Check sheet for the modelled part. Datum: model origin and axes. Units: mm. A direction names the side the tool comes from. Round coordinates to 2 decimals unless told otherwise and drop trailing zeros. Write each loop counter-clockwise with the first axis right and the second up, starting at its lowest first coordinate (ties: lowest second). Pieces come first, ordered by that corner, then holes.
Item 1: Release check for a two-part mould opening along Z. For faces 6 (the cylindrical face through (-27.101, 13.479, 31.486)), 7 (the flat face through (-40, 6, 24)), 8 (the flat face through (34, 0, 21)) record: pulls with the +Z half, pulls with the -Z half, needs draft (parallel to the pull), parting line crosses it, or undercut.
Item 2: Section check D-D, the plane y = 16.75. Record the cut outline in (x, z).
Item 3: Section check C-C, the plane y = 4. Record the cut outline in (x, z), plus the area to 3 significant figures.
Item 4: Depth check by flat-ended pin: pin 1 (3.5 mm diameter, centred on x = -37, z = 19, fed in from +Y); pin 2 (4 mm diameter, centred on x = 4.5, y = 8, fed in from -Z); pin 3 (12.5 mm diameter, centred on x = -37.24, z = 21.5, fed in from +Y); pin 4 (3.5 mm diameter, centred on x = 0, z = -43, fed in from +Y). Enter the tip coordinate at first touch or a pass-through.
Item 5: Section check B-B, the plane x = 0. Record the cut outline in (y, z), plus the area to 3 significant figures.
Item 6: Set-up check for faces 1 (the cylindrical face through (-43.54, 16.52, 6.46)), 2 (the cylindrical face through (-35.587, 11.916, 26.746)), 3 (the cylindrical face through (-40.9, 13.5, 7.9)), 4 (the cylindrical face through (-13.72, 13.48, -39.21)), 5 (the cylindrical face through (37.591, 5.916, 13.508)): record each of +Z, -Z, +X, -X, +Y, -Y from which the full face is reachable in a straight line by a thin tool's end or side.
Item 7: Material ranges on line 1 along X through (y, z) = (2.6, 21.5); line 2 along X through (y, z) = (15.25, 21.5); line 3 along X through (y, z) = (16, 22), recorded low to high.
Item 8: Section check A-A, the plane z = 21.5. State how many separate pieces and enclosed holes the cut face has, plus the area to 3 significant figures.
from build123d import *

# Parameters (mm, degrees)
SKETCH1_R             = 8
SKETCH1_R_2           = 3
BOSS_EXTRUDE1_DEPTH   = 6
BOSS_EXTRUDE1_2_DEPTH = 6
BOSS_EXTRUDE1_3_DEPTH = 6
BOSS_EXTRUDE3_START   = 18
SKETCH1_4_R           = 5.5
BOSS_EXTRUDE3_DEPTH   = 3
SKETCH1_3_R           = 8
SKETCH1_3_R_2         = 5.5
BOSS_EXTRUDE2_DEPTH   = 18
BOSS_EXTRUDE4_START   = 3
SKETCH2_R             = 8
BOSS_EXTRUDE4_DEPTH   = 3


with BuildPart() as part:
    # Sketch1 → Boss-Extrude1 (new body)
    with BuildSketch(Plane(origin=(0, 0, 0), x_dir=(1, 0, 0), z_dir=(0, 1, 0))):
        with Locations(Location((0, 43, 0), (0, 0, 270))):
            Circle(SKETCH1_R)
        with Locations(Location((0, 43, 0), (0, 0, 270))):
            Circle(SKETCH1_R_2, mode=Mode.SUBTRACT)
    extrude(amount=BOSS_EXTRUDE1_DEPTH)



with BuildPart() as body_2:
    # Sketch1 → Boss-Extrude1 2 (new body)
    with BuildSketch(Plane(origin=(0, 0, 0), x_dir=(1, 0, 0), z_dir=(0, 1, 0))):
        with Locations(Location((37.239092363, -21.5, 0), (0, 0, 270))):
            Circle(SKETCH1_R)
        with Locations(Location((37.239092363, -21.5, 0), (0, 0, 270))):
            Circle(SKETCH1_R_2, mode=Mode.SUBTRACT)
    extrude(amount=BOSS_EXTRUDE1_2_DEPTH)


with BuildPart() as body_3:
    # Sketch1 → Boss-Extrude1 3 (new body)
    with BuildSketch(Plane(origin=(0, 0, 0), x_dir=(1, 0, 0), z_dir=(0, 1, 0))):
        with Locations(Location((-37.239092363, -21.5, 0), (0, 0, 270))):
            Circle(SKETCH1_R)
        with Locations(Location((-37.239092363, -21.5, 0), (0, 0, 270))):
            Circle(SKETCH1_R_2, mode=Mode.SUBTRACT)
    extrude(amount=BOSS_EXTRUDE1_3_DEPTH)


with BuildPart() as body_4:
    # Sketch1<4> → Boss-Extrude3 (new body)
    with BuildSketch(Plane(origin=(0, 0, 0), x_dir=(1, 0, 0), z_dir=(0, 1, 0)).offset(BOSS_EXTRUDE3_START)):
        with BuildLine():
            ThreePointArc((14.941453584, 44.323995772), (0, 58), (-14.941453584, 44.323995772))
            ThreePointArc((-14.941453584, 44.323995772), (-16.147655157, 40.973517523), (-18.846153454, 38.65))
            ThreePointArc((-18.846153454, 38.65), (-37.239092363, 21.5), (-42.894958583, -3.003752345))
            ThreePointArc((-42.894958583, -3.003752345), (-43.557934635, -6.502479184), (-45.856433127, -9.222319513))
            ThreePointArc((-45.856433127, -9.222319513), (-50.229473419, -29), (-30.914979544, -35.101676259))
            ThreePointArc((-30.914979544, -35.101676259), (-27.410279478, -34.471038339), (-24.048805129, -35.646247655))
            ThreePointArc((-24.048805129, -35.646247655), (0, -43), (24.048805129, -35.646247655))
            ThreePointArc((24.048805129, -35.646247655), (27.410279478, -34.471038339), (30.914979544, -35.101676259))
            ThreePointArc((30.914979544, -35.101676259), (50.229473419, -29), (45.856433127, -9.222319513))
            ThreePointArc((45.856433127, -9.222319513), (43.557934635, -6.502479184), (42.894958583, -3.003752345))
            ThreePointArc((42.894958583, -3.003752345), (37.239092363, 21.5), (18.846153454, 38.65))
            ThreePointArc((18.846153454, 38.65), (16.147655157, 40.973517523), (14.941453584, 44.323995772))
        make_face()
        with Locations(Location((0, 43, 0), (0, 0, 270))):
            Circle(SKETCH1_4_R, mode=Mode.SUBTRACT)
        with Locations(Location((37.239092363, -21.5, 0), (0, 0, 270))):
            Circle(SKETCH1_4_R, mode=Mode.SUBTRACT)
        with Locations(Location((-37.239092363, -21.5, 0), (0, 0, 270))):
            Circle(SKETCH1_4_R, mode=Mode.SUBTRACT)
    extrude(amount=-BOSS_EXTRUDE3_DEPTH)


with BuildPart() as part_1:
    add(part.part)

    add(body_2.part)  # Boss-Extrude2 merges body 2

    add(body_3.part)  # Boss-Extrude2 merges body 3

    add(body_4.part)  # Boss-Extrude2 merges body 4
    # Sketch1<3> → Boss-Extrude2 (add)
    # profile 1 of 3: a face of its own
    with BuildSketch(Plane(origin=(0, 0, 0), x_dir=(1, 0, 0), z_dir=(0, 1, 0))):
        with Locations(Location((-37.239092363, -21.5, 0), (0, 0, 270))):
            Circle(SKETCH1_3_R)
        with Locations(Location((-37.239092363, -21.5, 0), (0, 0, 270))):
            Circle(SKETCH1_3_R_2, mode=Mode.SUBTRACT)
    # profile 2 of 3: a face of its own
    with BuildSketch(Plane(origin=(0, 0, 0), x_dir=(1, 0, 0), z_dir=(0, 1, 0))):
        with Locations(Location((37.239092363, -21.5, 0), (0, 0, 270))):
            Circle(SKETCH1_3_R)
        with Locations(Location((37.239092363, -21.5, 0), (0, 0, 270))):
            Circle(SKETCH1_3_R_2, mode=Mode.SUBTRACT)
    # profile 3 of 3: a face of its own
    with BuildSketch(Plane(origin=(0, 0, 0), x_dir=(1, 0, 0), z_dir=(0, 1, 0))):
        with Locations(Location((0, 43, 0), (0, 0, 270))):
            Circle(SKETCH1_3_R)
        with Locations(Location((0, 43, 0), (0, 0, 270))):
            Circle(SKETCH1_3_R_2, mode=Mode.SUBTRACT)
    extrude(amount=BOSS_EXTRUDE2_DEPTH)

    # Sketch2 → Boss-Extrude4 (add)
    with BuildSketch(Plane.XZ.offset(-15).offset(BOSS_EXTRUDE4_START)):
        with BuildLine():
            ThreePointArc((-39.902287054, 2.794188228), (-34.641016151, -20), (-17.531305538, -35.953488372))
            ThreePointArc((-17.531305538, -35.953488372), (-13.676307972, -39.272799119), (-11.953162867, -44.059196617))
            ThreePointArc((-11.953162867, -44.059196617), (0, -55), (11.953162867, -44.059196617))
            ThreePointArc((11.953162867, -44.059196617), (13.676307972, -39.272799119), (17.531305538, -35.953488372))
            ThreePointArc((17.531305538, -35.953488372), (34.641016151, -20), (39.902287054, 2.794188228))
            ThreePointArc((39.902287054, 2.794188228), (40.8493957, 7.792369426), (44.132964974, 11.67785561))
            ThreePointArc((44.132964974, 11.67785561), (47.631397208, 27.5), (32.179802107, 32.381341007))
            ThreePointArc((32.179802107, 32.381341007), (27.173087728, 31.480429693), (22.370981516, 33.159300144))
            ThreePointArc((22.370981516, 33.159300144), (0, 40), (-22.370981516, 33.159300144))
            ThreePointArc((-22.370981516, 33.159300144), (-27.173087728, 31.480429693), (-32.179802107, 32.381341007))
            ThreePointArc((-32.179802107, 32.381341007), (-47.631397208, 27.5), (-44.132964974, 11.67785561))
            ThreePointArc((-44.132964974, 11.67785561), (-40.8493957, 7.792369426), (-39.902287054, 2.794188228))
        make_face()
        with Locations(Location((0, -43, 0), (0, 0, 270))):
            Circle(SKETCH2_R, mode=Mode.SUBTRACT)
        with Locations(Location((37.239092363, 21.5, 0), (0, 0, 270))):
            Circle(SKETCH2_R, mode=Mode.SUBTRACT)
        with Locations(Location((-37.239092363, 21.5, 0), (0, 0, 270))):
            Circle(SKETCH2_R, mode=Mode.SUBTRACT)
    extrude(amount=-BOSS_EXTRUDE4_DEPTH)


solid = part_1.part
Values found:
1. face 6: pulls with the +Z half
1. face 7: undercut
1. face 8: needs draft
2. outline: (-45.86, 9.22) arc R7 cw to (-42.89, 3) arc R43 ccw to (-18.85, -38.65) arc R7 cw to (-14.94, -44.32) arc R15 ccw to (14.94, -44.32) arc R7 cw to (18.85, -38.65) arc R43 ccw to (42.89, 3) arc R7 cw to (45.86, 9.22) arc R15 ccw to (30.91, 35.1) arc R7 cw to (24.05, 35.65) arc R43 ccw to (-24.05, 35.65) arc R7 cw to (-30.91, 35.1) arc R15 ccw to start; hole circle Ø11 at (-37.24, 21.5); hole circle Ø11 at (0, -43); hole circle Ø11 at (37.24, 21.5)
3. outline: circle Ø16 at (-37.24, 21.5); circle Ø16 at (0, -43); circle Ø16 at (37.24, 21.5); hole circle Ø6 at (-37.24, 21.5); hole circle Ø6 at (0, -43); hole circle Ø6 at (37.24, 21.5)
3. area: 518 mm2
4. pin 1: stops at y = 6
4. pin 2: stops at z = -50.6
4. pin 3: stops at y = 18
4. pin 4: passes through
5. outline: (0, -51) - (12, -51) - (12, -55) - (15, -55) - (15, -58) - (18, -58) - (18, -48.5) - (6, -48.5) - (6, -46) - (0, -46) - close; (0, -40) - (6, -40) - (6, -37.5) - (18, -37.5) - (18, 43) - (15, 43) - (15, 40) - (12, 40) - (12, -35) - (0, -35) - close
5. area: 612 mm2
6. face 1: -X, +Y, -Y
6. face 2: +Y
6. face 3: -X, -Y
6. face 4: -Z, -X, -Y
6. face 5: -Y
7. line 1: x = -45.24 to -40.24, -34.24 to -29.24, 29.24 to 34.24, 40.24 to 45.24
7. line 2: x = -52.24 to -42.74, -31.74 to 31.74, 42.74 to 52.24
7. line 3: x = -52.23 to -42.72, -31.76 to 31.76, 42.72 to 52.23
8. separate pieces: 3
8. enclosed holes: 0
8. area: 657 mm2
